from build123d import *

# Parameters (mm, degrees)
SKETCH1_R           = 4.1
SKETCH1_R_2         = 1.6
BOSS_EXTRUDE1_DEPTH = 5
CHAMFER1_SIZE       = 1.7
CHAMFER2_SIZE       = 1.7


with BuildPart() as part:
    # Sketch1 → Boss-Extrude1 (new body)
    with BuildSketch(Plane(origin=(0, 0, 0), x_dir=(1, 0, 0), z_dir=(0, 1, 0))):
        with BuildLine():
            Line((-20.432418055, 3.512858569), (-7.567581945, 11.778442321))
            ThreePointArc((-7.567581945, 11.778442321), (0, 14), (7.567581945, 11.778442321))
            Line((7.567581945, 11.778442321), (20.432418055, 3.512858569))
            ThreePointArc((20.432418055, 3.512858569), (22.350852961, 0), (20.432418055, -3.512858569))
            Line((20.432418055, -3.512858569), (7.567581945, -11.778442321))
            ThreePointArc((7.567581945, -11.778442321), (0, -14), (-7.567581945, -11.778442321))
            Line((-7.567581945, -11.778442321), (-20.432418055, -3.512858569))
            ThreePointArc((-20.432418055, -3.512858569), (-22.350852961, 0), (-20.432418055, 3.512858569))
        make_face()
        with Locations(Location((0, 0, 0), (0, 0, 270))):
            Circle(SKETCH1_R, mode=Mode.SUBTRACT)
        with Locations(Location((-18.175426481, 0, 0), (0, 0, 270))):
            Circle(SKETCH1_R_2, mode=Mode.SUBTRACT)
        with Locations(Location((18.175426481, 0, 0), (0, 0, 270))):
            Circle(SKETCH1_R_2, mode=Mode.SUBTRACT)
        with Locations(Location((8, 0, 0), (0, 0, 270))):
            Circle(SKETCH1_R_2, mode=Mode.SUBTRACT)
        with Locations(Location((0, 8, 0), (0, 0, 270))):
            Circle(SKETCH1_R_2, mode=Mode.SUBTRACT)
        with Locations(Location((-8, 0, 0), (0, 0, 270))):
            Circle(SKETCH1_R_2, mode=Mode.SUBTRACT)
        with Locations(Location((0, -8, 0), (0, 0, 270))):
            Circle(SKETCH1_R_2, mode=Mode.SUBTRACT)
    extrude(amount=BOSS_EXTRUDE1_DEPTH)

    # Chamfer1
    chamfer1_edges = [part.edges().sort_by_distance(p)[0] for p in [
        (0, 5, -9.6),
        (8, 5, -1.6),
        (-8, 5, -1.6),
        (0, 5, 6.4),
    ]]
    chamfer(chamfer1_edges, length=CHAMFER1_SIZE)

    # Chamfer2
    chamfer2_edges = [part.edges().sort_by_distance(p)[0] for p in [
        (-18.175426481, 0, -1.6),
        (18.175426481, 0, -1.6),
    ]]
    chamfer(chamfer2_edges, length=CHAMFER2_SIZE)


solid = part.part
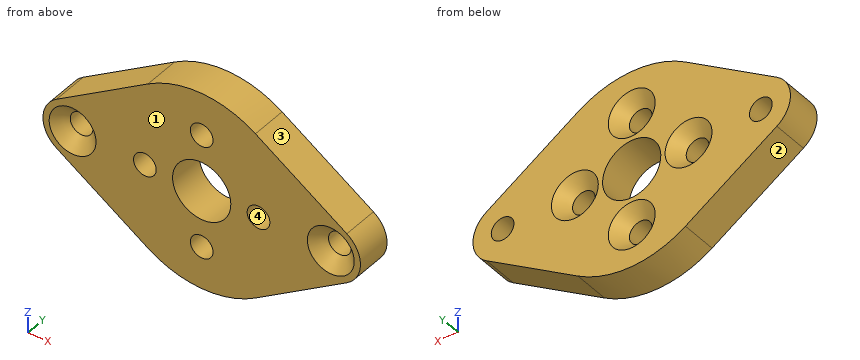
Model file for the job. Use its own axes, mm. Face numbers are marked on the shaded views. Give positions to 0.01 mm unless a question says otherwise; leave off trailing zeros. Loops run counter-clockwise (first coordinate to the right, second up) from the corner with the lowest first, then second, coordinate; pieces in that order, holes last. Notation, with made-up numbers: (12, -13) -> (68, -13) arc R23 ccw to (68, 12) -> close; hole circle Ø5 at (29.25, 26). An arc over 180 degrees is marked (long way). Use a Markdown table: item, result. Add a question column.
(1) Wall check: line 1 along X through (y, z) = (2.8, 0); line 2 along X through (y, z) = (4.1, 2); line 3 along X through (y, z) = (2.15, -1). Give the ranges that are in metal, low to high.
(2) Slice it at B-B on y = 1. List the corners of the cut face in (x, z), and give its area (3 significant figures).
(3) Slice it at A-A on x = 0. List the corners of the cut face in (y, z).
(4) Slice it at C-C on z = -8. List the corners of the cut face in (x, y), and give its area (3 significant figures).
(5) Mould opens along X. For the marked faces 1, 2, 3 and 4 say: +X half, -X half, draft (parallel to the pull), parting line (faces both ways), or undercut.
(6) Drop flat-ended pins along their axis: pin 1 Ø5 at (x, z) = (18.18, 0) entering from -Y; pin 2 Ø4 at (x, z) = (8, 0) entering from -Y; pin 3 Ø1.5 at (y, z) = (2, 9.5) entering from +X; pin 4 Ø4 at (x, z) = (0, -8) entering from +Y. Give the stop position or say it passes through.
(7) Slice it at D-D on x = -8. List the corners of the cut face in (y, z).
Filled sheet:
| question | item | result |
|---|---|---|
| 1 | line 1 | -22.35 to -19.78, -16.58 to -9.6, -6.4 to -4.1, 4.1 to 6.4, 9.6 to 16.58, 19.78 to 22.35 |
| 1 | line 2 | -21.84 to -9.33, -6.67 to -3.58, 3.58 to 6.67, 9.33 to 21.84 |
| 1 | line 3 | -22.23 to -19.42, -16.93 to -9.25, -6.75 to -3.98, 3.98 to 6.75, 9.25 to 16.93, 19.42 to 22.23 |
| 2 | outline | (-20.43, -3.51) -> (-7.57, -11.78) arc R14 ccw to (7.57, -11.78) -> (20.43, -3.51) arc R4.18 ccw to (20.43, 3.51) -> (7.57, 11.78) arc R14 ccw to (-7.57, 11.78) -> (-20.43, 3.51) arc R4.18 ccw to start; hole circle Ø4.6 at (-18.18, 0); hole circle Ø3.2 at (-8, 0); hole circle Ø8.2 at (0, 0); hole circle Ø3.2 at (0, -8); hole circle Ø3.2 at (0, 8); hole circle Ø3.2 at (8, 0); hole circle Ø4.6 at (18.18, 0) |
| 2 | area | 696 mm2 |
| 3 | outline | (0, -14) -> (5, -14) -> (5, -11.3) -> (3.3, -9.6) -> (0, -9.6) -> close; (0, -6.4) -> (3.3, -6.4) -> (5, -4.7) -> (5, -4.1) -> (0, -4.1) -> close; (0, 4.1) -> (5, 4.1) -> (5, 4.7) -> (3.3, 6.4) -> (0, 6.4) -> close; (0, 9.6) -> (3.3, 9.6) -> (5, 11.3) -> (5, 14) -> (0, 14) -> close |
| 4 | outline | (-13.45, 0) -> (-1.6, 0) -> (-1.6, 3.3) -> (-3.3, 5) -> (-13.45, 5) -> close; (1.6, 0) -> (13.45, 0) -> (13.45, 5) -> (3.3, 5) -> (1.6, 3.3) -> close |
| 4 | area | 116 mm2 |
| 5 | face 1 | draft |
| 5 | face 2 | -X half |
| 5 | face 3 | +X half |
| 5 | face 4 | undercut |
| 6 | pin 1 | y = 0.8 |
| 6 | pin 2 | y = 0 |
| 6 | pin 3 | x = 12.28 |
| 6 | pin 4 | y = 3.7 |
| 7 | outline | (0, -11.5) -> (5, -11.5) -> (5, -3.3) -> (3.3, -1.6) -> (0, -1.6) -> close; (0, 1.6) -> (3.3, 1.6) -> (5, 3.3) -> (5, 11.5) -> (0, 11.5) -> close |
